The listing builds one solid part. Answer for the finished solid, in the listing's coordinates (mm). Give positions to 0.01 mm unless a question says otherwise; leave off trailing zeros. Write each loop counter-clockwise with the first axis right and the second up, starting at its lowest first coordinate (ties: lowest second). Pieces come first, ordered by that corner, then holes. Notation, with made-up numbers: M 66,-19 L 91,-19 A6 ccw 91,-9 Z; hole C 55.5,28.25 d11. An arc over 180 degrees is marked long. Answer as a JSON object with one key per item and string values.
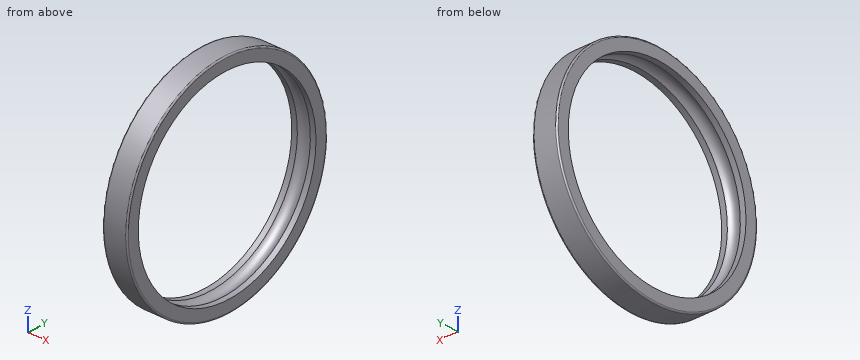
```python
from build123d import *


with BuildPart() as part:
    # Schizzo1 → Rivoluzione1 (revolve)
    with BuildSketch(Plane.XY, mode=Mode.PRIVATE) as rivoluzione1_sk:
        with BuildLine():
            Line((0, 79), (0, 70.975))
            Line((0, 70.975), (4.183737549, 70.975))
            ThreePointArc((4.183737549, 70.975), (9, 72.997), (13.816262451, 70.975))
            Line((13.816262451, 70.975), (18, 70.975))
            Line((18, 70.975), (18, 79))
            ThreePointArc((18, 79), (17.707106781, 79.707106781), (17, 80))
            Line((17, 80), (1, 80))
            ThreePointArc((1, 80), (0.292893219, 79.707106781), (0, 79))
        make_face()
    revolve(rivoluzione1_sk.sketch.rotate(Axis((200, 0, 0), (-1, 0, 0)), 270), axis=Axis((200, 0, 0), (-1, 0, 0)))


solid = part.part
```
1. Consider line 1 along Y through (x, z) = (14.9, 0) (3 decimals); line 2 along Y through (x, z) = (10, 45.5); line 3 along Z through (x, y) = (3, -18). Determine where each line is inside the solid, lowest interval first.
Verdict:
{"line 1": "y = -80 to -70.975, 70.975 to 80", "line 2": "y = -65.8 to -56.99, 56.99 to 65.8", "line 3": "z = -77.95 to -68.65, 68.65 to 77.95"}
2. Flat-ended cylindrical pins translate along their axes: pin 1 (4 mm diameter, centred on x = 12.5, z = -10.5, fed in from +Y); pin 2 (8 mm diameter, centred on x = 3, y = 12, fed in from +Z); pin 3 (8 mm diameter, centred on x = 9, y = -36, fed in from -Z). Find the tip coordinate at first contact, or state that the pin passes through.
Verdict:
{"pin 1": "stops at y = 79.55", "pin 2": "stops at z = 79.6", "pin 3": "stops at z = -73.32"}
3. A cutting plane is placed at A-A, the plane z = 0. Give the vertices of the cut face in (x, y) (3 decimals).
Verdict:
{"outline": "M 0,-79 A1 ccw 1,-80 L 17,-80 A1 ccw 18,-79 L 18,-70.975 L 13.816,-70.975 A6.747 cw 4.184,-70.975 L 0,-70.975 Z; M 0,70.975 L 4.184,70.975 A6.747 cw 13.816,70.975 L 18,70.975 L 18,79 A1 ccw 17,80 L 1,80 A1 ccw 0,79 Z"}
4. A cutting plane is placed at C-C, the plane x = 10.75. Give the vertices of the cut face in (y, z).
Verdict:
{"outline": "C 0,0 d160; hole C 0,0 d145.53"}
